For this review, take the finished solid that the model builds, in its own axes (mm). A direction names the side the tool comes from. Coordinates: 2 decimals unless noted, no trailing zeros. Order: outer loops, then holes, each group sorted by start corner. A loop starts at its lowest first (then second) coordinate and runs counter-clockwise, first axis right, second up.
from build123d import *

# Parameters (mm, degrees)
CROQUIS2_R                 = 1.5
CROQUIS2_R_2               = 12.5
CROQUIS2_W                 = 14
CROQUIS2_H                 = 6.4
CROQUIS2_W_2               = 15.2
CROQUIS2_H_2               = 24.4
SALIENTE_EXTRUIR1_DEPTH    = 13
CROQUIS3_R                 = 4
CORTAR_EXTRUIR1_DEPTH      = 30
CROQUIS4_W                 = 13
CROQUIS4_H                 = 25
CORTAR_EXTRUIR2_DEPTH      = 18
CORTAR_EXTRUIR3_DEPTH      = 63.491392709
CORTAR_EXTRUIR3_DEPTH_BACK = 63.491392709
CROQUIS5_R                 = 4.25


with BuildPart() as part:
    # Croquis2 → Saliente-Extruir1 (new body)
    # profile 1 of 2: a face of its own
    with BuildSketch(Plane.XY):
        with BuildLine():
            Line((-41.366340939, 30.306283288), (-41.366340939, 19.306283288))
            Line((-41.366340939, 19.306283288), (-41.366340939, -17.693716712))
            Line((-41.366340939, -17.693716712), (-41.366340939, -28.693716712))
            Line((-41.366340939, -28.693716712), (-13.366340939, -28.693716712))
            ThreePointArc((-13.366340939, -28.693716712), (-10.693254692, -27.919188273), (-8.848320971, -25.835560677))
            Line((-8.848320971, -25.835560677), (-4.921298265, -17.551872747))
            ThreePointArc((-4.921298265, -17.551872747), (-3.076364545, -15.468245151), (-0.403278298, -14.693716712))
            Line((-0.403278298, -14.693716712), (29.233659061, -14.693716712))
            ThreePointArc((29.233659061, -14.693716712), (32.769192967, -13.229250618), (34.233659061, -9.693716712))
            Line((34.233659061, -9.693716712), (34.233659061, 11.306283288))
            ThreePointArc((34.233659061, 11.306283288), (32.769192967, 14.841817194), (29.233659061, 16.306283288))
            Line((29.233659061, 16.306283288), (-0.403278298, 16.306283288))
            ThreePointArc((-0.403278298, 16.306283288), (-3.076364545, 17.080811727), (-4.921298265, 19.164439323))
            Line((-4.921298265, 19.164439323), (-8.848320971, 27.448127253))
            ThreePointArc((-8.848320971, 27.448127253), (-10.693254692, 29.531754849), (-13.366340939, 30.306283288))
            Line((-13.366340939, 30.306283288), (-41.366340939, 30.306283288))
        make_face()
        with Locations(Location((-38.366340939, -14.693716712, 0), (0, 0, 180))):
            Circle(CROQUIS2_R, mode=Mode.SUBTRACT)
        with Locations(Location((-7.366340939, -14.693716712, 0), (0, 0, 180))):
            Circle(CROQUIS2_R, mode=Mode.SUBTRACT)
        with Locations(Location((-24.366340939, 0.806283288, 0), (0, 0, 180))):
            Circle(CROQUIS2_R_2, mode=Mode.SUBTRACT)
        with Locations(Location((-38.366340939, 16.306283288, 0), (0, 0, 180))):
            Circle(CROQUIS2_R, mode=Mode.SUBTRACT)
        with Locations(Location((-7.366340939, 16.306283288, 0), (0, 0, 180))):
            Circle(CROQUIS2_R, mode=Mode.SUBTRACT)
        with Locations((1.703659061, 0.906283288)):
            Rectangle(CROQUIS2_W, CROQUIS2_H, mode=Mode.SUBTRACT)
        with Locations((22.133659061, 0.906283288)):
            Rectangle(CROQUIS2_W_2, CROQUIS2_H_2, mode=Mode.SUBTRACT)
    # profile 2 of 2: a face of its own
    with BuildSketch(Plane.XY):
        with BuildLine():
            Line((-41.366340939, 30.306283288), (-41.366340939, 19.306283288))
            Line((-41.366340939, 19.306283288), (-41.366340939, -17.693716712))
            Line((-41.366340939, -17.693716712), (-41.366340939, -28.693716712))
            Line((-41.366340939, -28.693716712), (-13.366340939, -28.693716712))
            ThreePointArc((-13.366340939, -28.693716712), (-10.693254692, -27.919188273), (-8.848320971, -25.835560677))
            Line((-8.848320971, -25.835560677), (-4.921298265, -17.551872747))
            ThreePointArc((-4.921298265, -17.551872747), (-3.076364545, -15.468245151), (-0.403278298, -14.693716712))
            Line((-0.403278298, -14.693716712), (29.233659061, -14.693716712))
            ThreePointArc((29.233659061, -14.693716712), (32.769192967, -13.229250618), (34.233659061, -9.693716712))
            Line((34.233659061, -9.693716712), (34.233659061, 11.306283288))
            ThreePointArc((34.233659061, 11.306283288), (32.769192967, 14.841817194), (29.233659061, 16.306283288))
            Line((29.233659061, 16.306283288), (-0.403278298, 16.306283288))
            ThreePointArc((-0.403278298, 16.306283288), (-3.076364545, 17.080811727), (-4.921298265, 19.164439323))
            Line((-4.921298265, 19.164439323), (-8.848320971, 27.448127253))
            ThreePointArc((-8.848320971, 27.448127253), (-10.693254692, 29.531754849), (-13.366340939, 30.306283288))
            Line((-13.366340939, 30.306283288), (-41.366340939, 30.306283288))
        make_face()
        with Locations(Location((-38.366340939, -14.693716712, 0), (0, 0, 180))):
            Circle(CROQUIS2_R, mode=Mode.SUBTRACT)
        with Locations(Location((-7.366340939, -14.693716712, 0), (0, 0, 180))):
            Circle(CROQUIS2_R, mode=Mode.SUBTRACT)
        with Locations(Location((-24.366340939, 0.806283288, 0), (0, 0, 180))):
            Circle(CROQUIS2_R_2, mode=Mode.SUBTRACT)
        with Locations(Location((-38.366340939, 16.306283288, 0), (0, 0, 180))):
            Circle(CROQUIS2_R, mode=Mode.SUBTRACT)
        with Locations(Location((-7.366340939, 16.306283288, 0), (0, 0, 180))):
            Circle(CROQUIS2_R, mode=Mode.SUBTRACT)
        with Locations((1.703659061, 0.906283288)):
            Rectangle(CROQUIS2_W, CROQUIS2_H, mode=Mode.SUBTRACT)
        with Locations((22.133659061, 0.906283288)):
            Rectangle(CROQUIS2_W_2, CROQUIS2_H_2, mode=Mode.SUBTRACT)
    extrude(amount=SALIENTE_EXTRUIR1_DEPTH)

    # Croquis3 → Cortar-Extruir1 (cut)
    with BuildSketch(Plane.ZY.offset(41.366340939)):
        with Locations(Location((6.5, 23.806283288, 0), (0, 0, 270))):
            Circle(CROQUIS3_R)
        with Locations(Location((6.5, -22.193716712, 0), (0, 0, 270))):
            Circle(CROQUIS3_R)
    extrude(amount=-CORTAR_EXTRUIR1_DEPTH, mode=Mode.SUBTRACT)

    # Croquis4 → Cortar-Extruir2 (cut)
    with BuildSketch(Plane.ZY.offset(41.366340939)):
        with Locations((6.5, 0.806283288)):
            Rectangle(CROQUIS4_W, CROQUIS4_H)
    extrude(amount=-CORTAR_EXTRUIR2_DEPTH, mode=Mode.SUBTRACT)

    # Croquis5 → Cortar-Extruir3 (cut, two sides: drawn at the far end of the back side and taken through both)
    with BuildSketch(Plane(origin=(0, 16.306283288, 0), x_dir=(1, 0, 0), z_dir=(0, 1, 0)).offset(-CORTAR_EXTRUIR3_DEPTH_BACK)):
        with Locations(Location((22.133659061, -6.5, 0), (0, 0, 270))):
            Circle(CROQUIS5_R)
        with Locations(Location((1.703659061, -6.5, 0), (0, 0, 270))):
            Circle(CROQUIS5_R)
    extrude(amount=CORTAR_EXTRUIR3_DEPTH + CORTAR_EXTRUIR3_DEPTH_BACK, mode=Mode.SUBTRACT)


solid = part.part
1. Take a section at C-C, the plane z = 6.5. Give the number of separate pieces and of enclosed holes in the cut face, plus the area to 3 significant figures.
Answer below:
separate pieces: 3
enclosed holes: 4
area: 1,390 mm2
2. Take a section at A-A, the plane x = -32. Give the boundary of the cut face in (y, z), plus the area to 3 significant figures.
Answer below:
outline: (-28.69, 0) - (-11.69, 0) - (-11.69, 13) - (-28.69, 13) - close; (13.31, 0) - (30.31, 0) - (30.31, 13) - (13.31, 13) - close; hole circle Ø8 at (-22.19, 6.5); hole circle Ø8 at (23.81, 6.5)
area: 341 mm2
3. The part is to be moulded in two halves that separate along X. For faces 1 (the face through (-10.73, -27.94, 6.41)), 2 (the face through (19.548, 14.684, 3.127)), 3 (the face through (-11.366, 24, 7)), say which applies: +X half, -X half, draft (parallel to the pull), parting line (faces both ways), or undercut.
Answer below:
face 1: +X half
face 2: undercut
face 3: -X half
4. Take a section at D-D, the plane x = 20.5. Give the boundary of the cut face in (y, z), plus the area to 3 significant figures.
Answer below:
outline: (-14.69, 0) - (-11.29, 0) - (-11.29, 2.58) - (-14.69, 2.58) - close; (-14.69, 10.42) - (-11.29, 10.42) - (-11.29, 13) - (-14.69, 13) - close; (13.11, 0) - (16.31, 0) - (16.31, 2.58) - (13.11, 2.58) - close; (13.11, 10.42) - (16.31, 10.42) - (16.31, 13) - (13.11, 13) - close
area: 34.0 mm2
5. Machinability: for faces 4 (the face through (-32, -11.694, 6)), 5 (the face through (14.534, 1, 6)), 6 (the face through (-12, -5, 0)), which of the approach directions +Z, -Z, +X, -X, +Y, -Y give a long, thin tool a straight path to every point of the face, cutting with its end or side? Answer none if there is none.
Answer below:
face 4: +Z, -Z, -X
face 5: +Z, -Z
face 6: -Z, +X, -X, +Y, -Y
6. To check wall thickness, follow L1, parallel to Y at x = 18, z = 5; L2, parallel to Y at x = -7, z = 8.5; L3, parallel to Y at x = -32, z = 2. State the ranges of each line that lie inside material, in increasing order.
Answer below:
L1: y = -14.69 to -11.29, 13.11 to 16.31
L2: y = -21.94 to -16.15, -13.24 to 14.85, 17.76 to 23.55
L3: y = -28.69 to -11.69, 13.31 to 30.31
7. Take a section at B-B, the plane y = 9. Give the boundary of the cut face in (x, z), plus the area to 3 significant figures.
Answer below:
outline: (-14.93, 0) - (14.53, 0) - (14.53, 13) - (-14.93, 13) - close; (29.73, 0) - (34.23, 0) - (34.23, 13) - (29.73, 13) - close; hole circle Ø8.5 at (1.7, 6.5)
area: 385 mm2
8. Clearance check with flat-ended pins moving along their axes: pin 1 Ø4 at (y, z) = (-18, 5.5) entering from +X; pin 2 Ø7.5 at (x, z) = (1.7, 6.5) entering from +Y; pin 3 Ø3 at (y, z) = (-0.5, 6) entering from -X; pin 4 Ø5 at (y, z) = (-22.19, 6.5) entering from -X. State where each tip first meets the part, or that it passes through.
Answer below:
pin 1: stops at x = -3.77
pin 2: passes through
pin 3: stops at x = -12.19
pin 4: stops at x = -11.37
